```python
from build123d import *

# Parameters (mm, degrees)
SKETCH_2_W               = 180
SKETCH_2_H               = 180
EXTRUDE_1_DEPTH          = 8.5
CHAMFER_1_SIZE           = 20
SKETCH_4_R               = 5.5
CUT_EXTRUDE_1_DEPTH      = 8.5
MIRROR_2_COPY_1_SKETCH_R = 5.5
MIRROR_2_COPY_1_DEPTH    = 8.5
SKETCH_5_R               = 20
CUT_EXTRUDE_2_DEPTH      = 1089.345359905


with BuildPart() as part:
    # 草图1 → 旋转1 (revolve)
    with BuildSketch(Plane.XY, mode=Mode.PRIVATE) as revolve_1_sk:
        with BuildLine():
            ThreePointArc((922.973468016, 268.381765717), (922.094788359, 266.260445373), (919.973468016, 265.381765717))
            Line((919.973468016, 265.381765717), (922.973468016, 265.381765717))
            Line((922.973468016, 265.381765717), (992.973468016, 265.381765717))
            Line((992.973468016, 265.381765717), (992.973468016, 313.381765717))
            Line((992.973468016, 313.381765717), (959.973468016, 313.381765717))
            Line((959.973468016, 313.381765717), (925.973468016, 313.381765717))
            ThreePointArc((925.973468016, 313.381765717), (923.852147672, 312.50308606), (922.973468016, 310.381765717))
            Line((922.973468016, 310.381765717), (922.973468016, 268.381765717))
        make_face()
        with BuildLine():
            Line((959.973468016, 313.381765717), (992.973468016, 313.381765717))
            Line((992.973468016, 313.381765717), (992.973468016, 316.581765717))
            Line((992.973468016, 316.581765717), (962.973468016, 316.581765717))
            Line((962.973468016, 316.581765717), (962.973468016, 316.381765717))
            ThreePointArc((962.973468016, 316.381765717), (962.094788359, 314.260445373), (959.973468016, 313.381765717))
        make_face()
    revolve(revolve_1_sk.sketch.rotate(Axis((992.973468016, 256.881765717, 0), (0, 1, 0)), 270), axis=Axis((992.973468016, 256.881765717, 0), (0, 1, 0)))

    # 草图2 → 凸台-拉伸1 (add)
    with BuildSketch(Plane.XZ.offset(-265.381765717)):
        with Locations((992.973468016, 0)):
            Rectangle(SKETCH_2_W, SKETCH_2_H)
    extrude(amount=EXTRUDE_1_DEPTH)

    # 倒角1
    chamfer_1_edges = [part.edges().sort_by_distance(p)[0] for p in [
        (1082.973468016, 261.131765717, -90),
        (1082.973468016, 261.131765717, 90),
        (902.973468016, 261.131765717, 90),
        (902.973468016, 261.131765717, -90),
    ]]
    chamfer(chamfer_1_edges, length=CHAMFER_1_SIZE)

    # 草图4 → 切除-拉伸1 (cut)
    with BuildSketch(Plane.XZ.offset(-256.881765717)):
        with Locations(Location((1062.973468016, 70, 0), (0, 0, 270))):
            Circle(SKETCH_4_R)
    cut_extrude_1 = extrude(amount=-CUT_EXTRUDE_1_DEPTH, mode=Mode.SUBTRACT)

    # 镜向1: 切除-拉伸1 across plane
    add(cut_extrude_1.mirror(Plane.XY), mode=Mode.SUBTRACT)

    # 镜向2: 切除-拉伸1 across plane
    add(cut_extrude_1.mirror(Plane.ZY.offset(-992.973468016)), mode=Mode.SUBTRACT)

    # 镜向2 copy 1 sketch → 镜向2 copy 1 (cut)
    with BuildSketch(Plane(origin=(1985.946936032, 256.881765717, 0), x_dir=(-1, 0, 0), z_dir=(0, -1, 0))):
        with Locations(Location((1062.973468016, 70, 0), (0, 0, 270))):
            Circle(MIRROR_2_COPY_1_SKETCH_R)
    extrude(amount=-MIRROR_2_COPY_1_DEPTH, mode=Mode.SUBTRACT)

    # 草图5 → 切除-拉伸2 (cut, through all)
    with BuildSketch(Plane.XZ.offset(-256.881765717)):
        with Locations(Location((992.973468016, 0, 0), (0, 0, 270))):
            Circle(SKETCH_5_R)
    extrude(amount=-CUT_EXTRUDE_2_DEPTH, mode=Mode.SUBTRACT)


solid = part.part
```
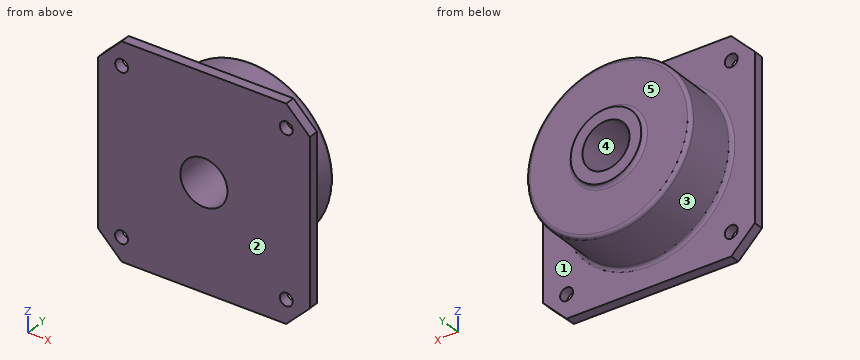
Input: part model. Units: mm. Frame: model coordinates. Face numbers are marked on the shaded views. A direction names the side the tool comes from. Give positions to 0.01 mm unless a question says otherwise; leave off trailing zeros. Write each loop counter-clockwise with the first axis right and the second up, starting at its lowest first coordinate (ties: lowest second). Pieces come first, ordered by that corner, then holes. Notation, with made-up numbers: (22, 13) - (59, 13) arc R24 cw to (59, 47) - close; hole circle Ø1 at (57.5, 66). An arc over 180 degrees is marked (long way). Write item = value, one per line. Start each with the question number.
1) Draft query along X for the marked faces 3, 4 and 5. Return one class per face: pulls with the +X half, pulls with the -X half, needs draft (parallel to the pull), parting line crosses it, or undercut.
2) Cut plane B-B (y = 290.5). Return loops of the section in (x, z).
3) Material intervals for L1, parallel to X at y = 285, z = 0; L2, parallel to Y at x = 947.5, z = 17.5; L3, parallel to X at y = 286, z = 3, sorted ascending. Write a range as [from, to].
4) Cut plane A-A (z = 0). Return loops of the section in (x, y), and give its area (3 significant figures).
5) Reachability of the marked faces 1 and 2 from +Z, -Z, +X, -X, +Y, -Y: full face, straight path, thin tool, end or side. Return the list, or none.
6) Pin query (flat end, axial travel): pin 1 (2 mm diameter, centred on x = 934.5, y = 274.5, fed in from -Z); pin 2 (10 mm diameter, centred on y = 290, z = -40.5, fed in from +X); pin 3 (2 mm diameter, centred on x = 986.5, y = 306, fed in from -Z). Return the tip coordinate at first contact, or that it passes through.
Answers follow:
q1.face_3 = parting line crosses it
q1.face_4 = undercut
q1.face_5 = needs draft
q2.outline = circle Ø140 at (992.97, 0); hole circle Ø40 at (992.97, 0)
q3.L1 = [922.97, 972.97], [1012.97, 1062.97]
q3.L2 = [256.88, 313.38]
q3.L3 = [923.04, 973.2], [1012.75, 1062.91]
q4.outline = (902.97, 256.88) - (972.97, 256.88) - (972.97, 316.58) - (962.97, 316.58) - (962.97, 316.38) arc R3 cw to (959.97, 313.38) - (925.97, 313.38) arc R3 ccw to (922.97, 310.38) - (922.97, 268.38) arc R3 cw to (919.97, 265.38) - (902.97, 265.38) - close; (1012.97, 256.88) - (1082.97, 256.88) - (1082.97, 265.38) - (1065.97, 265.38) arc R3 cw to (1062.97, 268.38) - (1062.97, 310.38) arc R3 ccw to (1059.97, 313.38) - (1025.97, 313.38) arc R3 cw to (1022.97, 316.38) - (1022.97, 316.58) - (1012.97, 316.58) - close
q4.area = 6,060 mm^2
q5.face_1 = +Y
q5.face_2 = +Z, -Z, +X, -X, -Y
q6.pin_1 = -39.96
q6.pin_2 = 1053.3
q6.pin_3 = -69.79
